Geometry check sheet. Reference: the model listing, model coordinates, mm. A direction names the side the tool comes from. Give positions to 0.01 mm unless a question says otherwise; leave off trailing zeros. Write each loop counter-clockwise with the first axis right and the second up, starting at its lowest first coordinate (ties: lowest second). Pieces come first, ordered by that corner, then holes. Notation, with made-up numbers: M 1.5,21.25 L 43.5,21.25 A25 ccw 43.5,44.25 Z; hole C 28.5,58.25 d5. An arc over 180 degrees is marked long. One line per item, written item: value. Start each with the question number.
1. Gauge pin test, flat ends, axial feed: pin 1 (2.5 mm diameter, centred on x = -1, z = 29, fed in from -Y); pin 2 (10 mm diameter, centred on x = -11, z = 45, fed in from -Y); pin 3 (12 mm diameter, centred on y = 280, z = 14, fed in from -X); pin 4 (23.5 mm diameter, centred on x = -30, y = 341.5, fed in from +Z). Record the tip position at first contact, or that the pin passes through.
2. Tool access check on faces 1 (the face through (-3, 253.6, 26.8)), 2 (the face through (-25, 254, 0)). Record the directions out of +Z, -Z, +X, -X, +Y, -Y that give a thin tool (end or side, any length) a straight path to the whole face; none if there is none.
3. Cross-section at B-B on x = -19.5. Record the cut outline in (y, z).
4. Cross-section at A-A on y = 232.5. Record the cut outline in (x, z), then the cut area to 3 significant figures.
5. Scan lines: line 1 (Z direction, x = -30, y = 224); line 2 (X direction, y = 121.5, z = 7). Record each from-to range of solid material in increasing order.
Autodesk Inventor part; units mm, degrees
ref_plane "YZ Plane" through (0, 0, 0) normal (1, 0, 0) x (0, 1, 0)
ref_plane "XZ Plane" through (0, 0, 0) normal (0, 1, 0) x (-1, 0, 0)
ref_plane "XY Plane" through (0, 0, 0) normal (0, 0, 1) x (1, 0, 0)
sketch "Sketch1" plane through (0, 0, 0) normal (0, 1, 0) x (-1, 0, 0)
  line L0 (0, 0) -> (50, 0)
  line L1 (50, 0) -> (50, 3)
  line L2 (0, 0) -> (0, 50)
  line L3 (0, 50) -> (3, 50)
  line L4 (3, 50) -> (3, 3)
  line L5 (3, 3) -> (50, 3)
  dimension "d0" = 50
  dimension "d1" = 3
  dimension "d2" = 50
  dimension "d3" = 3
extrude "Extrusion1" add sketch "Sketch1" along normal blind 514.4008
sketch "Sketch2" plane through (-3, 0, 3) normal (-1, 0, 0) x (0, 0, 1)
  line L0 (0, 514.4008) -> (47, 514.4008)
  line L1 (0, 0) -> (47, 0)
  line L2 (47, 0) -> (47, 514.4008)
  line L3 (0, 0) -> (0, 514.4008)
  line L4 (-3, 0) -> (-3, 514.4008)
  line L5 (-3, 0) -> (0, 0)
  line L6 (-3, 514.4008) -> (0, 514.4008)
  line L7 (12.7, 498.4008) -> (34.3, 498.4008) construction
  line L8 (12.7, 501.5758) -> (34.3, 501.5758)
  line L9 (12.7, 495.2258) -> (34.3, 495.2258)
  arc A0 (12.7, 501.5758) -> (12.7, 495.2258) centre (12.7, 498.4008) ccw
  arc A1 (34.3, 495.2258) -> (34.3, 501.5758) centre (34.3, 498.4008) ccw
  line L10 (12.7, 19.175) -> (34.3, 19.175)
  line L11 (34.3, 12.825) -> (12.7, 12.825)
  line L12 (12.7, 16) -> (34.3, 16) construction
  arc A2 (12.7, 19.175) -> (12.7, 12.825) centre (12.7, 16) ccw
  arc A3 (34.3, 12.825) -> (34.3, 19.175) centre (34.3, 16) ccw
  line L13 (12.7, 136.6002) -> (34.3, 136.6002) construction
  line L14 (12.7, 139.7752) -> (34.3, 139.7752)
  line L15 (12.7, 133.4252) -> (34.3, 133.4252)
  arc A4 (12.7, 139.7752) -> (12.7, 133.4252) centre (12.7, 136.6002) ccw
  arc A5 (34.3, 133.4252) -> (34.3, 139.7752) centre (34.3, 136.6002) ccw
  line L16 (12.7, 377.8006) -> (34.3, 377.8006) construction
  line L17 (12.7, 380.9756) -> (34.3, 380.9756)
  line L18 (12.7, 374.6256) -> (34.3, 374.6256)
  arc A6 (12.7, 380.9756) -> (12.7, 374.6256) centre (12.7, 377.8006) ccw
  arc A7 (34.3, 374.6256) -> (34.3, 380.9756) centre (34.3, 377.8006) ccw
  line L19 (12.7, 257.2004) -> (34.3, 257.2004) construction
  line L20 (12.7, 260.3754) -> (34.3, 260.3754)
  line L21 (12.7, 254.0254) -> (34.3, 254.0254)
  arc A8 (12.7, 260.3754) -> (12.7, 254.0254) centre (12.7, 257.2004) ccw
  arc A9 (34.3, 254.0254) -> (34.3, 260.3754) centre (34.3, 257.2004) ccw
  dimension "d58" = 12.7
  dimension "d59" = 12.7
  dimension "d60" = 3.175
  dimension "d61" = 6.35
  dimension "d62" = 6.35
  dimension "d63" = 3.175
  dimension "d70" = 16
  dimension "d73" = 16
  dimension "d74" = 3.175
  dimension "d75" = 6.35
  dimension "d76" = 3.175
  dimension "d77" = 6.35
  dimension "d78" = 3.175
  dimension "d79" = 6.35
  dimension "d80" = 482.4008
  dimension "d81" = 120.6002
  dimension "d82" = 120.6002
  dimension "d83" = 120.6002
extrude "Extrusion3" cut sketch "Sketch2" against normal blind 3 contours L8 A1 L9 A0 | L10 A3 L11 A2 | L14 A5 L15 A4 | L17 A7 L18 A6 | L20 A9 L21 A8
equation "\"d73\" = d70"
equation "\"d81\" = 0.25 * d80"
equation "\"d82\" = d81"
equation "\"d83\" = d82"
properties part number "26in Angle Channel" material "Aluminum 6061"
Report:
1. pin 1: stops at y = 0
1. pin 2: passes through
1. pin 3: stops at x = -3
1. pin 4: stops at z = 3
2. face 1: +Z, -X, +Y, -Y
2. face 2: -Z, +X, -X, +Y, -Y
3. outline: M 0,0 L 514.4,0 L 514.4,3 L 0,3 Z
4. outline: M -50,0 L 0,0 L 0,50 L -3,50 L -3,3 L -50,3 Z
4. area: 291 mm^2
5. line 1: z = 0 to 3
5. line 2: x = -3 to 0
